Here's how the part is built. I have some questions about the finished solid (model axes, mm). Face numbers are marked on the shaded views. Give positions to 0.01 mm unless a question says otherwise; leave off trailing zeros. Write each loop counter-clockwise with the first axis right and the second up, starting at its lowest first coordinate (ties: lowest second). Pieces come first, ordered by that corner, then holes. Notation, with made-up numbers: (-26.5, 89.5) -> (1.5, 89.5) arc R27 cw to (1.5, 125.5) -> close; hole circle Ø7 at (-32.5, -11). An arc over 180 degrees is marked (long way). Use one line per item in the form item = value.
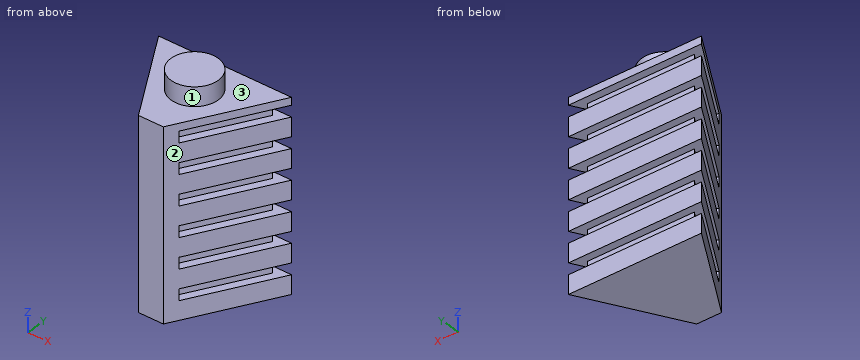
```python
from build123d import *

# Parameters (mm, degrees)
F1_DEPTH  = 127
F2_W      = 89.5684185014
F2_H      = 63.5
F3_DEPTH  = 215.9
F4_R      = 15.875
F5_DEPTH  = 139.7
F6_W      = 88.9
F6_H      = 7.62
F7_DEPTH  = 5.08
F8_W      = 63.5
F8_H      = 7.62
F9_DEPTH  = 5.08
F10_W     = 63.5
F10_H     = 7.62
F11_DEPTH = 5.08


with BuildPart() as f1:
    # F0 (on Top) → F1 (new body)
    with BuildSketch(Plane.XY):
        Polygon((44.45, 25.6632194655), (-44.45, 25.6632194655), (0, -51.326438931), align=None)
    extrude(amount=F1_DEPTH)

    # F2 (on Top) → F3 (intersect)
    with BuildSketch(Plane.XY):
        with Locations((-0.2493504435, -5.1686391234)):
            Rectangle(F2_W, F2_H)
    extrude(amount=F3_DEPTH, mode=Mode.INTERSECT)

    # F4 (on Top) → F5 (join)
    with BuildSketch(Plane.XY):
        Circle(F4_R)
    extrude(amount=F5_DEPTH)

    # F6 (on face) → F7 (cut)
    with BuildSketch(Plane(origin=(0, 25.6632194655, 0), x_dir=(-1, 0, 0), z_dir=(0, 1, 0))):
        with Locations((0, 16.51)):
            Rectangle(F6_W, F6_H)
        with Locations((0, 36.83)):
            Rectangle(F6_W, F6_H)
        with Locations((0, 57.15)):
            Rectangle(F6_W, F6_H)
        with Locations((0, 77.47)):
            Rectangle(F6_W, F6_H)
        with Locations((0, 97.79)):
            Rectangle(F6_W, F6_H)
        with Locations((0, 118.11)):
            Rectangle(F6_W, F6_H)
    extrude(amount=-F7_DEPTH, mode=Mode.SUBTRACT)

    # F8 (on face) → F9 (cut)
    with BuildSketch(Plane(origin=(22.225, -12.8316097327, 0), x_dir=(0.5, 0.8660254038, 0), z_dir=(0.8660254038, -0.5, 0))):
        with Locations((12.7, 16.51)):
            Rectangle(F8_W, F8_H)
        with Locations((12.7, 36.83)):
            Rectangle(F8_W, F8_H)
        with Locations((12.7, 57.15)):
            Rectangle(F8_W, F8_H)
        with Locations((12.7, 77.47)):
            Rectangle(F8_W, F8_H)
        with Locations((12.7, 97.79)):
            Rectangle(F8_W, F8_H)
        with Locations((12.7, 118.11)):
            Rectangle(F8_W, F8_H)
    extrude(amount=-F9_DEPTH, mode=Mode.SUBTRACT)

    # F10 (on face) → F11 (cut)
    with BuildSketch(Plane(origin=(-22.225, -12.8316097327, 0), x_dir=(0.5, -0.8660254038, 0), z_dir=(-0.8660254038, -0.5, 0))):
        with Locations((-12.7, 16.51)):
            Rectangle(F10_W, F10_H)
        with Locations((-12.7, 36.83)):
            Rectangle(F10_W, F10_H)
        with Locations((-12.7, 57.15)):
            Rectangle(F10_W, F10_H)
        with Locations((-12.7, 77.47)):
            Rectangle(F10_W, F10_H)
        with Locations((-12.7, 97.79)):
            Rectangle(F10_W, F10_H)
        with Locations((-12.7, 118.11)):
            Rectangle(F10_W, F10_H)
    extrude(amount=-F11_DEPTH, mode=Mode.SUBTRACT)


solid = f1.part
```
Q1. If we mould it in two halves opening along X, with no side actions, what happens to the marked faces 1, 2 and 3? For each: +X half, -X half, draft (parallel to the pull), parting line (faces both ways), or undercut.
Result set:
face_1 = parting line
face_2 = +X half
face_3 = draft
Q2. I want a section at B-B, the plane z = 110. Write out the boundary of the cut face in (x, y), and give its area (3 significant figures).
Result set:
outline = (-44.45, 25.66) -> (-8.32, -36.92) -> (8.32, -36.92) -> (44.45, 25.66) -> close
area = 3,300 mm2
Q3. If I drill on line 1 along Z through (x, y) = (0, -16.5); line 2 along Y through (x, z) = (1, 128.5); line 3 along Y through (x, z) = (35.5, 79), over which ranges is the centre line in solid material (lowest first)? Write a range as from..to.
Result set:
line_1 = 0..127
line_2 = -15.84..15.84
line_3 = 20.32..20.58
Q4. I want a section at C-C, the plane x = -10.5. Count the separate pieces of the cut face and the enclosed holes in it, and give its area (3 significant figures).
Result set:
separate_pieces = 1
enclosed_holes = 6
area = 7,310 mm2
Q5. Will these pins go through, and if not, where does the flat tip stop? pin 1 Ø1.5 at (y, z) = (14, 32) entering from +X; pin 2 Ø2 at (x, z) = (24, 14.5) entering from -Y; pin 3 Ø1 at (x, z) = (0, 118.5) entering from +Y.
Result set:
pin_1 = 38.15
pin_2 = -1.33
pin_3 = 20.58
